Input: part model. Units: mm. Frame: model coordinates. Face numbers are marked on the shaded views. Coordinates: 2 decimals unless noted, no trailing zeros. Loops run counter-clockwise (first coordinate to the right, second up) from the corner with the lowest first, then second, coordinate; pieces in that order, holes last.
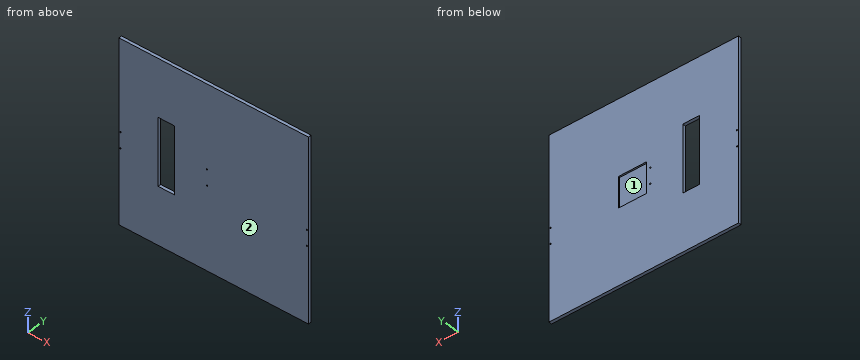
```python
from build123d import *

# Parameters (mm, degrees)
SKETCH_1_W             = 620
SKETCH_1_H             = 580
EXTRUDE_1_DEPTH        = 10
HOLE_WIZARD_M5_1_D     = 4.2
HOLE_WIZARD_M5_1_DEPTH = 12.2
HOLE_WIZARD_M5_1_TIP   = 1.2618073
SKETCH_5_W             = 54
SKETCH_5_H             = 214
CUT_EXTRUDE_1_DEPTH    = 425.617474911
HOLE_WIZARD_M5_2_D     = 4.2
SKETCH_10_W            = 92
SKETCH_10_H            = 98
CUT_EXTRUDE_2_DEPTH    = 5


with BuildPart() as part:
    # 草图1 → 凸台-拉伸1 (new body)
    with BuildSketch(Plane(origin=(0, 0, 0), x_dir=(1, 0, 0), z_dir=(0, 1, 0))):
        Rectangle(SKETCH_1_W, SKETCH_1_H)
    extrude(amount=EXTRUDE_1_DEPTH)

    # M5 螺纹孔1
    with Locations(Plane(origin=(0, 10, 0), x_dir=(1, 0, 0), z_dir=(0, 1, 0))):
        with Locations((-305, 50), (-305, 0), (305, 0), (305, 50)):
            Hole(HOLE_WIZARD_M5_1_D / 2, depth=HOLE_WIZARD_M5_1_DEPTH)
            with Locations((0, 0, -(HOLE_WIZARD_M5_1_DEPTH + HOLE_WIZARD_M5_1_TIP / 2))):  # 118° drill point
                Cone(0, HOLE_WIZARD_M5_1_D / 2, HOLE_WIZARD_M5_1_TIP, mode=Mode.SUBTRACT)

    # 草图5 → 切除-拉伸1 (cut, through all)
    with BuildSketch(Plane.XZ):
        with Locations((-155, 0)):
            Rectangle(SKETCH_5_W, SKETCH_5_H)
    extrude(amount=-CUT_EXTRUDE_1_DEPTH, mode=Mode.SUBTRACT)

    # M5 螺纹孔2 (through all)
    with Locations(Plane(origin=(0, 0, 0), x_dir=(-1, 0, 0), z_dir=(0, -1, 0))):
        with Locations((21.6, -25), (21.6, 25)):
            Hole(HOLE_WIZARD_M5_2_D / 2)

    # 草图10 → 切除-拉伸2 (cut)
    with BuildSketch(Plane(origin=(0, 10, 0), x_dir=(1, 0, 0), z_dir=(0, 1, 0))):
        with Locations((36.9, 0)):
            Rectangle(SKETCH_10_W, SKETCH_10_H)
    extrude(amount=-CUT_EXTRUDE_2_DEPTH, mode=Mode.SUBTRACT)


solid = part.part
```
Item 1: Section query A-A (z = 34). Output: boundary loops of the cut face in (x, y), then the cut area to 3 significant figures.
Result:
outline: (-310, 0) - (-182, 0) - (-182, 10) - (-310, 10) - close; (-128, 0) - (310, 0) - (310, 10) - (82.9, 10) - (82.9, 5) - (-9.1, 5) - (-9.1, 10) - (-128, 10) - close
area: 5,200 mm2
Item 2: Mould query, pull axis Z, two halves, no side actions, for the marked faces 1 and 2. Classes: +Z half, -Z half, draft (parallel to the pull), parting line (faces both ways), or undercut.
Result:
face 1: undercut
face 2: draft
Item 3: Section query B-B (y = 6.5). Count the separate pieces of the cut face and the enclosed holes in it, then the cut area to 3 significant figures.
Result:
separate pieces: 1
enclosed holes: 8
area: 339,000 mm2
Item 4: Line query: L1, parallel to X at y = 3.75, z = -25; L2, parallel to Z at x = 305, y = 7.5; L3, parallel to X at y = 3, z = -102.5. Output: solid intervals per line, ascending.
Result:
L1: x = -310 to -182, -128 to -23.7, -19.5 to 310
L2: z = -290 to -52.1, -47.9 to -2.1, 2.1 to 290
L3: x = -310 to -182, -128 to 310
Item 5: Contact query for flat-ended pins moving along their axis: P1, Ø4, axis at x = -21.6, z = -25, coming from the -Y side; P2, Ø5, axis at x = 229.5, z = -34.5, coming from the -Y side. Output: stop coordinate, or through.
Result:
P1: passes through
P2: stops at y = 0
Item 6: Section query C-C (x = 60.5). Output: boundary loops of the cut face in (y, z), then the cut area to 3 significant figures.
Result:
outline: (0, -290) - (10, -290) - (10, -49) - (5, -49) - (5, 49) - (10, 49) - (10, 290) - (0, 290) - close
area: 5,310 mm2
